Autodesk Inventor part; units mm, degrees
ref_plane "Plano de trabalho1" through (0, 0, 0) normal (0, 0, 1) x (1, 0, 0)
ref_plane "YZ Plane" through (0, 0, 0) normal (1, 0, 0) x (0, 1, 0)
ref_plane "XZ Plane" through (0, 0, 0) normal (0, 1, 0) x (-1, 0, 0)
ref_plane "Plano de trabalho1" through (0, 0, 0) normal (0, 0, 1) x (1, 0, 0)
sketch "Esboço1" plane through (0, 0, 0) normal (0, 0, 1) x (1, 0, 0)
  arc A0 (-40, -30) -> (-30, -40) centre (-30, -30) ccw
  line L0 (30, -40) -> (-30, -40)
  arc A1 (30, -40) -> (40, -30) centre (30, -30) ccw
  line L1 (40, 30) -> (40, -30)
  arc A2 (40, 30) -> (30, 40) centre (30, 30) ccw
  line L2 (-30, 40) -> (30, 40)
  arc A3 (-30, 40) -> (-40, 30) centre (-30, 30) ccw
  line L3 (-40, -30) -> (-40, 30)
  circle A4 centre (0, 0) radius 5
  circle A5 centre (0, 0) radius 5
  circle A6 centre (30, 30) radius 2
  circle A7 centre (30, -30) radius 2
  circle A8 centre (-30, -30) radius 2
  circle A9 centre (-30, 30) radius 2
  point P0 (0, 0)
  dimension "d0" = 10
  dimension "d3" = 4
  dimension "d4" = 4
  dimension "d5" = 4
  dimension "d6" = 4
extrude "Extrusão1" add sketch "Esboço1" along normal blind 12
equation "\"d3\" = d6"
equation "\"d4\" = d6"
equation "\"d5\" = d6"
properties part number "corpo_01a"
The listing builds one solid part. Answer for the finished solid, in the listing's coordinates (mm). Give positions to 0.01 mm unless a question says otherwise; leave off trailing zeros. Order: outer loops, then holes, each group sorted by start corner. A loop starts at its lowest first (then second) coordinate and runs counter-clockwise, first axis right, second up. Notation, with made-up numbers: (35, 41.5) - (70, 41.5) arc R18 ccw to (70, 61.5) - close; hole circle Ø7 at (-2, -7.5). An arc over 180 degrees is marked (long way). Answer in a Markdown table with one row per item. Add a question column.
Q1. Given P1, Ø4.5, axis at x = 30, y = -30, coming from the -Z side, flat-ended and moving along its own axis, determine where the tip first touches the part or whether it passes through.
Q2. For a pull along Y with two mould halves and no side action, classify faces 1 (the flat face through (8, 1, 0)), 2 (the cylindrical face through (37.15, -36.99, 5.92)), 3 (the cylindrical face through (-29.077, -28.226, 5.916)), 4 (the flat face through (0, 40, 6)) as released by +Y, released by -Y, zero draft, split by the parting line, or undercut.
Q3. The part is cut by section D-D (x = 29). Determine the outline of the cut face in (y, z), then the cut area to 3 significant figures.
Q4. Find the intervals of material crossed by line 1 along Y through (x, z) = (-30, 4.5); line 2 along Y through (x, z) = (0, 3.5); line 3 along X through (y, z) = (-28.5, 5), in increasing order. Write a range as [from, to].
Q5. The part is cut by section A-A (y = 0). Determine the outline of the cut face in (x, z), then the cut area to 3 significant figures.
Q6. The part is cut by section B-B (z = 3.75). Determine the outline of the cut face in (x, y), then the cut area to 3 significant figures.
Determined:
| question | item | result |
|---|---|---|
| 1 | P1 | stops at z = 0 |
| 2 | face 1 | zero draft |
| 2 | face 2 | released by -Y |
| 2 | face 3 | undercut |
| 2 | face 4 | released by +Y |
| 3 | outline | (-40, 0) - (-31.73, 0) - (-31.73, 12) - (-40, 12) - close; (-28.27, 0) - (28.27, 0) - (28.27, 12) - (-28.27, 12) - close; (31.73, 0) - (40, 0) - (40, 12) - (31.73, 12) - close |
| 3 | area | 877 mm² |
| 4 | line 1 | y = [-40, -32], [-28, 28], [32, 40] |
| 4 | line 2 | y = [-40, -5], [5, 40] |
| 4 | line 3 | x = [-40, -31.32], [-28.68, 28.68], [31.32, 40] |
| 5 | outline | (-40, 0) - (-5, 0) - (-5, 12) - (-40, 12) - close; (5, 0) - (40, 0) - (40, 12) - (5, 12) - close |
| 5 | area | 840 mm² |
| 6 | outline | (-40, -30) arc R10 ccw to (-30, -40) - (30, -40) arc R10 ccw to (40, -30) - (40, 30) arc R10 ccw to (30, 40) - (-30, 40) arc R10 ccw to (-40, 30) - close; hole circle Ø4 at (-30, -30); hole circle Ø4 at (-30, 30); hole circle Ø10 at (0, 0); hole circle Ø4 at (30, -30); hole circle Ø4 at (30, 30) |
| 6 | area | 6,190 mm² |
